Can you work these out from the model? Positions are in its coordinate system, mm. Coordinates: 2 decimals unless noted, no trailing zeros. Loops run counter-clockwise (first coordinate to the right, second up) from the corner with the lowest first, then second, coordinate; pieces in that order, holes last. Notation, with made-up numbers: M -20,0.25 L 13,0.25 A14 ccw 13,9.25 Z; hole C -32,56 d7. An arc over 180 degrees is marked long. Answer as a JSON object with one key per item and string values. Group by question number.
Item 1: If I drill on line 1 (Y direction, x = 0, z = 3.75) (3 decimals); line 2 (X direction, y = 15.5, z = 1) (3 decimals); line 3 (Y direction, x = -11.5, z = 2.75) (3 decimals), over which ranges is the centre line in solid material (lowest first)?
Item 2: Suppose I cut it at C-C (y = 0). Write out the boundary of the cut face in (x, z) (3 decimals).
Item 3: Suppose I cut it at D-D (x = -7.5). Count the separate pieces of the cut face and the enclosed holes in it, then the cut area to 3 significant figures.
Item 4: I'm going to push a flat-ended pin straight in: pin 1 Ø13.5 at (x, y) = (0, 0) entering from +Z. Where does the tip first touch, or does it pass through?
Item 5: Suppose I cut it at B-B (z = 4.5). Write out the boundary of the cut face in (x, y) (3 decimals).
Item 6: Suppose I cut it at A-A (x = 0). Write out the boundary of the cut face in (y, z) (3 decimals), then the cut area to 3 significant figures.
Item 7: We'd pull the mould along X, two halves only. Please class faces 1 (the flat face through (-15.875, 0, 3)), 2 (the flat face through (15.875, 0, 3)), 3 (the flat face through (0, 22.225, 3)), 4 (the cylindrical face through (-12.697, -15.735, 3.134)): +X half, -X half, draft (parallel to the pull), parting line (faces both ways), or undercut.
```python
from build123d import *

# Parameters (mm, degrees)
SKETCH1_W           = 31.75
SKETCH1_H           = 44.45
SKETCH1_R           = 3.175
SKETCH1_R_2         = 11.176
BOSS_EXTRUDE1_DEPTH = 6.35
CHAMFER1_SIZE       = 0.254


with BuildPart() as part:
    # Sketch1 → Boss-Extrude1 (new body)
    with BuildSketch(Plane.XY):
        Rectangle(SKETCH1_W, SKETCH1_H)
        with Locations((-9.525, 15.875)):
            Circle(SKETCH1_R, mode=Mode.SUBTRACT)
        with Locations((9.525, 15.875)):
            Circle(SKETCH1_R, mode=Mode.SUBTRACT)
        with Locations((-9.525, -15.875)):
            Circle(SKETCH1_R, mode=Mode.SUBTRACT)
        with Locations((9.525, -15.875)):
            Circle(SKETCH1_R, mode=Mode.SUBTRACT)
        Circle(SKETCH1_R_2, mode=Mode.SUBTRACT)
    extrude(amount=BOSS_EXTRUDE1_DEPTH)

    # Chamfer1
    chamfer1_edges = [part.edges().sort_by_distance(p)[0] for p in [
        (-15.875, 0, 6.35),
        (-12.7, 15.875, 0),
        (-12.7, 15.875, 6.35),
        (0, -22.225, 6.35),
        (6.35, 15.875, 0),
        (6.35, 15.875, 6.35),
        (-12.7, -15.875, 0),
        (-12.7, -15.875, 6.35),
        (6.35, -15.875, 0),
        (6.35, -15.875, 6.35),
        (-11.176, 0, 0),
        (-11.176, 0, 6.35),
        (15.875, 0, 6.35),
        (0, -22.225, 0),
        (-15.875, 0, 0),
        (0, 22.225, 0),
        (15.875, 0, 0),
        (0, 22.225, 6.35),
    ]]
    chamfer(chamfer1_edges, length=CHAMFER1_SIZE)


solid = part.part
```
From the geometry:
{
 "1": {"line 1": "-22.225 to -11.176, 11.176 to 22.225", "line 2": "-15.875 to -12.678, -6.372 to 6.372, 12.678 to 15.875", "line 3": "-22.225 to -18.361, -13.389 to 13.389, 18.361 to 22.225"},
 "2": {"outline": "M -15.875,0.254 L -15.621,0 L -11.43,0 L -11.176,0.254 L -11.176,6.096 L -11.43,6.35 L -15.621,6.35 L -15.875,6.096 Z; M 11.176,0.254 L 11.43,0 L 15.621,0 L 15.875,0.254 L 15.875,6.096 L 15.621,6.35 L 11.43,6.35 L 11.176,6.096 Z"},
 "3": {"separate pieces": "4", "enclosed holes": "0", "area": "114 mm2"},
 "4": {"pin 1": "through"},
 "5": {"outline": "M -15.875,-22.225 L 15.875,-22.225 L 15.875,22.225 L -15.875,22.225 Z; hole C -9.525,-15.875 d6.35; hole C -9.525,15.875 d6.35; hole C 0,0 d22.352; hole C 9.525,-15.875 d6.35; hole C 9.525,15.875 d6.35"},
 "6": {"outline": "M -22.225,0.254 L -21.971,0 L -11.43,0 L -11.176,0.254 L -11.176,6.096 L -11.43,6.35 L -21.971,6.35 L -22.225,6.096 Z; M 11.176,0.254 L 11.43,0 L 21.971,0 L 22.225,0.254 L 22.225,6.096 L 21.971,6.35 L 11.43,6.35 L 11.176,6.096 Z", "area": "140 mm2"},
 "7": {"face 1": "-X half", "face 2": "+X half", "face 3": "draft", "face 4": "undercut"}
}
